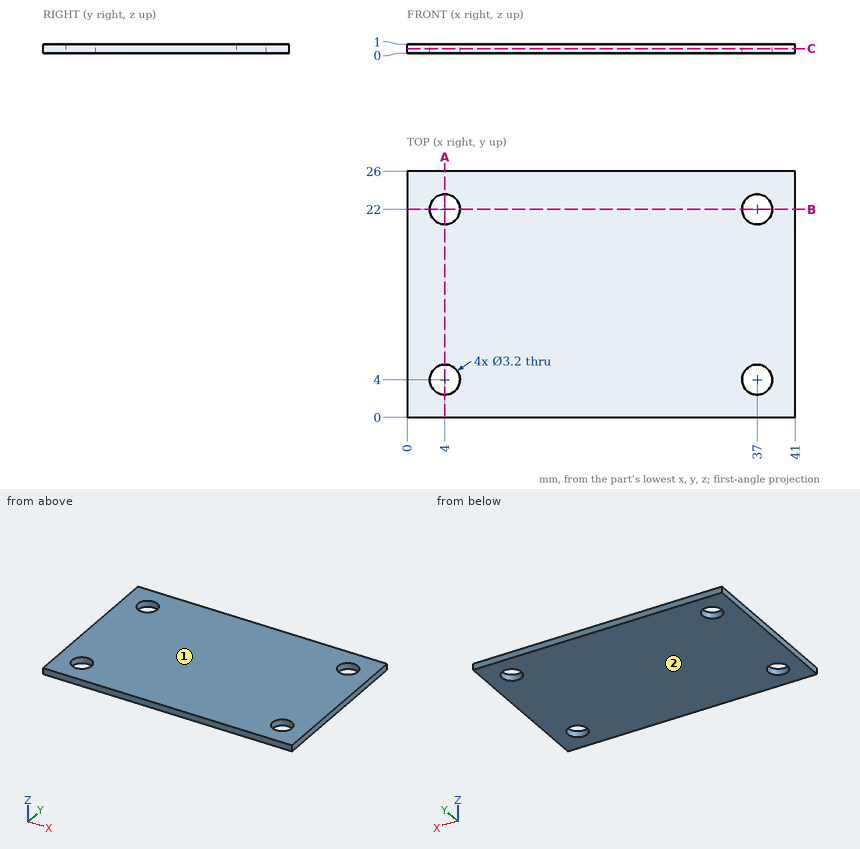
Job drawing, mm, ordinate dimensions from the low corner. One solid piece. Give positions to 0.01 mm unless a question says otherwise; leave off trailing zeros. Loops run counter-clockwise (first coordinate to the right, second up) from the corner with the lowest first, then second, coordinate; pieces in that order, holes last. Notation, with made-up numbers: M 27,-16.5 L 63,-16.5 A30 cw 63,21.5 Z; hole C -35.5,60 d9. An arc over 180 degrees is marked long. Answer in a Markdown table with one row per item. Add a question column.
Item 1: Band-saw the part on B-B on y = 22. Give the cut face in (x, z), then the cut area to 3 significant figures.
Item 2: Mould opens along Z. For the marked faces 1 and 2 say: +Z half, -Z half, draft (parallel to the pull), parting line (faces both ways), or undercut.
Item 3: Band-saw the part on A-A on x = 4. Give the cut face in (y, z), then the cut area to 3 significant figures.
Item 4: Probe probe 1 along Y at (x, z) = (4, 0.75); probe 2 along X at (y, z) = (22, 0.65); probe 3 along X at (y, z) = (20.75, 0.3). List the from-to ranges inside material, lowest first.
Item 5: Band-saw the part on C-C on z = 0.5. Give the cut face in (x, y), then the cut area to 3 significant figures.
Reply:
| question | item | result |
|---|---|---|
| 1 | outline | M 0,0 L 2.4,0 L 2.4,1 L 0,1 Z; M 5.6,0 L 35.4,0 L 35.4,1 L 5.6,1 Z; M 38.6,0 L 41,0 L 41,1 L 38.6,1 Z |
| 1 | area | 34.6 mm^2 |
| 2 | face 1 | +Z half |
| 2 | face 2 | -Z half |
| 3 | outline | M 0,0 L 2.4,0 L 2.4,1 L 0,1 Z; M 5.6,0 L 20.4,0 L 20.4,1 L 5.6,1 Z; M 23.6,0 L 26,0 L 26,1 L 23.6,1 Z |
| 3 | area | 19.6 mm^2 |
| 4 | probe 1 | y = 0 to 2.4, 5.6 to 20.4, 23.6 to 26 |
| 4 | probe 2 | x = 0 to 2.4, 5.6 to 35.4, 38.6 to 41 |
| 4 | probe 3 | x = 0 to 3, 5 to 36, 38 to 41 |
| 5 | outline | M 0,0 L 41,0 L 41,26 L 0,26 Z; hole C 4,4 d3.2; hole C 4,22 d3.2; hole C 37,4 d3.2; hole C 37,22 d3.2 |
| 5 | area | 1,030 mm^2 |
